Could you check a few things on this drawing? It's one solid part, dimensions in mm from its lowest x, y, z. A direction names the side the tool comes from. Give positions to 0.01 mm unless a question says otherwise; leave off trailing zeros. Loops run counter-clockwise (first coordinate to the right, second up) from the corner with the lowest first, then second, coordinate; pieces in that order, holes last. Notation, with made-up numbers: (89, 31.25) - (99, 31.25) arc R25 ccw to (99, 57.25) - close; hole circle Ø6 at (70, 83). An arc over 180 degrees is marked (long way). Return JSON: item names as keys, results as strings. Group by question number.
(1) If we section it at D-D (y = 49): Please give me the cut outline in (x, z), then the cut area to 3 significant figures.
(2) If we section it at A-A (z = 8): Please give me the cut outline in (x, y), then the cut area to 3 significant figures.
(3) If we section it at C-C (z = 23): Please give me the cut outline in (x, y).
(4) On a 3-axis mill with a long thin cutter (end or side, diameter ignored), from which of +Z, -Z, +X, -X, +Y, -Y can I reach the whole of each face in a straight line? I mean the marked faces 1 and 2. Say none if no direction works.
(5) For P1, Ø10, axis at y = 45.5, z = 23, coming from the +X side; P2, Ø3.5, axis at x = 5, y = 29.5, coming from the -Z side, each with a flat end and sliding along its axis, tell me the tip position at first contact or that it passes through.
(6) If we mould it in two halves opening along Y, with no side actions, what happens to the marked faces 3, 4 and 5? For each: released by +Y, released by -Y, zero draft, split by the parting line, or undercut.
(7) I need wall thicknesses on probe 1 along Y at (x, z) = (6.25, 10); probe 2 along Y at (x, z) = (3.5, 15); probe 3 along Z at (x, y) = (0.5, 66.5). Which ranges of each line are inside material? Lowest first, please. Write a range as [from, to].
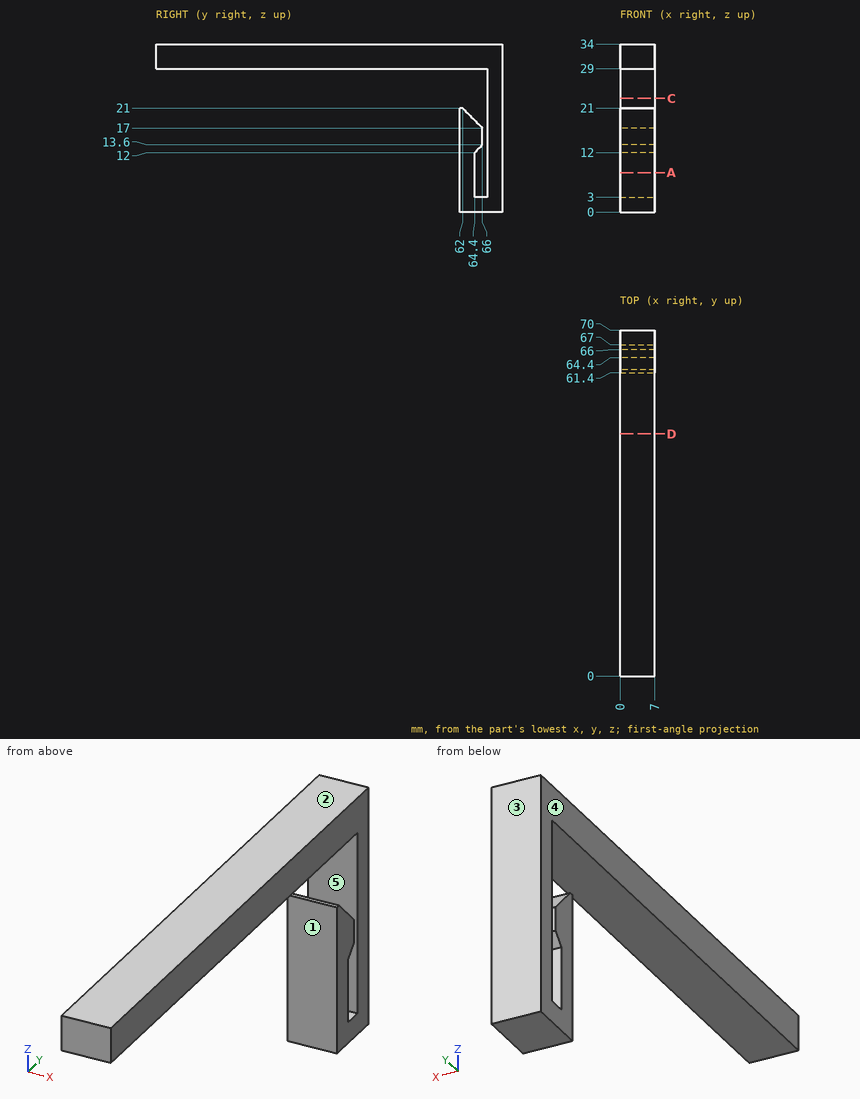
Values:
{
 "1": {"outline": "(0, 29) - (7, 29) - (7, 34) - (0, 34) - close", "area": "35.0 mm2"},
 "2": {"outline": "(0, 61.4) - (7, 61.4) - (7, 64.4) - (0, 64.4) - close; (0, 67) - (7, 67) - (7, 70) - (0, 70) - close", "area": "42.0 mm2"},
 "3": {"outline": "(0, 67) - (7, 67) - (7, 70) - (0, 70) - close"},
 "4": {"face 1": "-Z, +X, -X, -Y", "face 2": "+Z, +X, -X, +Y, -Y"},
 "5": {"P1": "through", "P2": "z = 29"},
 "6": {"face 3": "released by +Y", "face 4": "zero draft", "face 5": "undercut"},
 "7": {"probe 1": "[61.4, 64.4], [67, 70]", "probe 2": "[61.4, 66], [67, 70]", "probe 3": "[0, 3], [29, 34]"}
}
